Here's the drawing with two shaded views (mm, measured from the low corner). I have some questions. A direction names the side the tool comes from. Give positions to 0.01 mm unless a question says otherwise; leave off trailing zeros. Write each loop counter-clockwise with the first axis right and the second up, starting at its lowest first coordinate (ties: lowest second). Pieces come first, ordered by that corner, then holes. Notation, with made-up numbers: M 81,60 L 114,60 A9 cw 114,70 Z; hole C 84.25,87.5 d10. An arc over 180 degrees is marked long. Use one line per item in the form item = value. Start each with the question number.
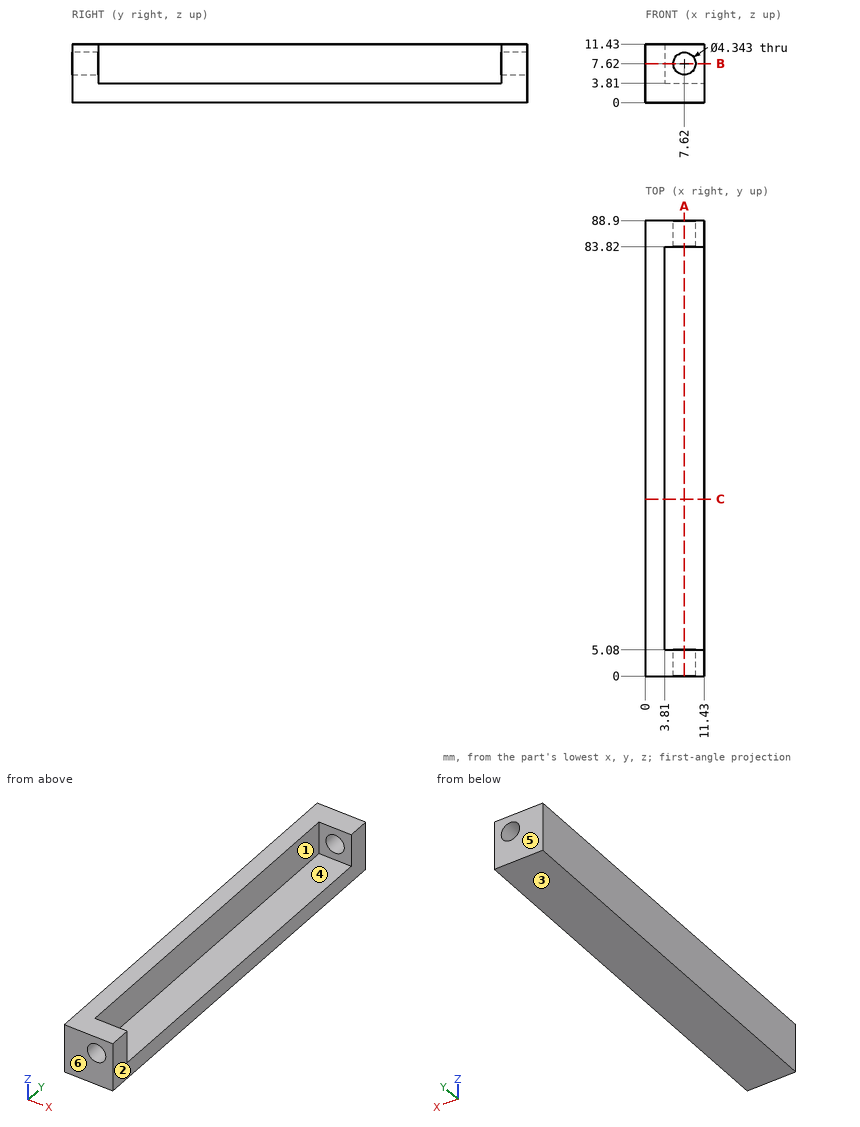
1) Will this pin go through, and if not, where does the flat tip stop? P1, Ø6, axis at x = 7, y = 51.5, coming from the +Z side.
2) Suppose I cut it at A-A, the plane x = 7.62. List the corners of the cut face in (y, z) for me.
3) Please list where these lines run through material, in increasing order: line 1 (X direction, y = 85, z = 7.62); line 2 (Y direction, x = 9.5, z = 9.75); line 3 (X direction, y = 27, z = 10).
4) Suppose I cut it at C-C, the plane y = 34.5. List the corners of the cut face in (x, z) for me.
5) Thinking about a two-plate mould opening in Y: for the marked faces 3, 4, 5 and 6, which applies, released by +Y, released by -Y, zero draft, split by the parting line, or undercut?
6) Suppose I cut it at B-B, the plane z = 7.62. List the corners of the cut face in (x, y) for me.
7) On a 3-axis mill with a long thin cutter (end or side, diameter ignored), from which of +Z, -Z, +X, -X, +Y, -Y can I reach the whole of each face in a straight line? I mean the marked faces 1 and 2. Say none if no direction works.
Checks:
q1.P1 = 3.81
q2.outline = M 0,0 L 88.9,0 L 88.9,5.45 L 83.82,5.45 L 83.82,3.81 L 5.08,3.81 L 5.08,5.45 L 0,5.45 Z; M 0,9.79 L 5.08,9.79 L 5.08,11.43 L 0,11.43 Z; M 83.82,9.79 L 88.9,9.79 L 88.9,11.43 L 83.82,11.43 Z
q3.line_1 = 0 to 5.45, 9.79 to 11.43
q3.line_2 = 0 to 5.08, 83.82 to 88.9
q3.line_3 = 0 to 3.81
q4.outline = M 0,0 L 11.43,0 L 11.43,3.81 L 3.81,3.81 L 3.81,11.43 L 0,11.43 Z
q5.face_3 = zero draft
q5.face_4 = undercut
q5.face_5 = released by +Y
q5.face_6 = released by -Y
q6.outline = M 0,0 L 5.45,0 L 5.45,5.08 L 3.81,5.08 L 3.81,83.82 L 5.45,83.82 L 5.45,88.9 L 0,88.9 Z; M 9.79,0 L 11.43,0 L 11.43,5.08 L 9.79,5.08 Z; M 9.79,83.82 L 11.43,83.82 L 11.43,88.9 L 9.79,88.9 Z
q7.face_1 = +Z, +X
q7.face_2 = +Z, -Z, +X, +Y, -Y
